from build123d import *

# Parameters (mm, degrees)
BOSS_EXTRUDE1_DEPTH = 3
SKETCH2_R           = 1.5
CUT_EXTRUDE1_DEPTH  = 3
CUT_EXTRUDE2_DEPTH  = 3
SKETCH5_W           = 18
SKETCH5_H           = 3
CUT_EXTRUDE3_DEPTH  = 3
CUT_EXTRUDE5_DEPTH  = 3


with BuildPart() as part:
    # Sketch1 → Boss-Extrude1 (new body)
    with BuildSketch(Plane.XY):
        with BuildLine():
            Line((3.868741846, 4.666984775), (3.868741846, -4.333015225))
            ThreePointArc((3.868741846, -4.333015225), (2.990062189, -6.454335569), (0.868741846, -7.333015225))
            Line((0.868741846, -7.333015225), (-29.131258154, -7.333015225))
            ThreePointArc((-29.131258154, -7.333015225), (-39.055484202, 1.438271074), (-31.570064658, 12.365037303))
            Line((-31.570064658, 12.365037303), (-13.143764854, 16.998769659))
            ThreePointArc((-13.143764854, 16.998769659), (-7.545321729, 14.563041923), (-8.476085741, 8.52905374))
            ThreePointArc((-8.476085741, 8.52905374), (-8.5954965, 7.981289437), (-8.131258154, 7.666984775))
            Line((-8.131258154, 7.666984775), (0.868741846, 7.666984775))
            ThreePointArc((0.868741846, 7.666984775), (2.990062189, 6.788305118), (3.868741846, 4.666984775))
        make_face()
    extrude(amount=BOSS_EXTRUDE1_DEPTH)

    # Sketch2 → Cut-Extrude1 (cut)
    with BuildSketch(Plane.XY.offset(3)):
        with Locations((-29.131258154, 2.666984775)):
            Circle(SKETCH2_R)
    extrude(amount=-CUT_EXTRUDE1_DEPTH, mode=Mode.SUBTRACT)

    # Sketch4 → Cut-Extrude2 (cut)
    with BuildSketch(Plane(origin=(0, 0, 0), x_dir=(-1, 0, 0), z_dir=(0, 0, -1))):
        with BuildLine():
            Line((30.632745307, 6.129616333), (16.185458015, 12.394336069))
            ThreePointArc((16.185458015, 12.394336069), (13.596850059, 11.433034125), (14.450350699, 8.806909749))
            Line((14.450350699, 8.806909749), (26.890771517, -0.370201523))
            ThreePointArc((26.890771517, -0.370201523), (32.402104849, 0.783943915), (30.632745307, 6.129616333))
        make_face()
    extrude(amount=-CUT_EXTRUDE2_DEPTH, mode=Mode.SUBTRACT)

    # Sketch5 → Cut-Extrude3 (cut)
    with BuildSketch(Plane.XY.offset(3)):
        with Locations((-8.131258154, -1.533015225)):
            Rectangle(SKETCH5_W, SKETCH5_H)
    extrude(amount=-CUT_EXTRUDE3_DEPTH, mode=Mode.SUBTRACT)

    # Sketch7 → Cut-Extrude5 (cut)
    with BuildSketch(Plane.XY.offset(3)):
        with BuildLine():
            Line((-14.631258154, -0.033015225), (-14.631258154, 3.966984775))
            ThreePointArc((-14.631258154, 3.966984775), (-14.338364936, 4.674091556), (-13.631258154, 4.966984775))
            Line((-13.631258154, 4.966984775), (-2.631258154, 4.966984775))
            ThreePointArc((-2.631258154, 4.966984775), (-1.924151373, 4.674091556), (-1.631258154, 3.966984775))
            Line((-1.631258154, 3.966984775), (-1.631258154, -0.033015225))
            Line((-1.631258154, -0.033015225), (-14.631258154, -0.033015225))
        make_face()
    extrude(amount=-CUT_EXTRUDE5_DEPTH, mode=Mode.SUBTRACT)


solid = part.part
Verification items for the finished model (mm, model axes). A direction names the side the tool comes from. Coordinates: 2 decimals unless noted, no trailing zeros. Order: outer loops, then holes, each group sorted by start corner. A loop starts at its lowest first (then second) coordinate and runs counter-clockwise, first axis right, second up. Notation, with made-up numbers: (74, -10) -> (86, -10) arc R16 ccw to (86, 20) -> close; hole circle Ø3 at (0.5, 37.25). An arc over 180 degrees is marked (long way). Put each result on its own line as item: value. Start each with the question number.
1. Go/stop test with flat-tipped pins: pin 1 Ø12 at (x, y) = (-29.13, 2.67) entering from -Z; pin 2 Ø1.5 at (x, z) = (-4, 1.5) entering from +Y. Record where each tip stops, or that it passes through.
2. Mould release check, pull along X, two halves, no side actions. Record for faces 3 (the flat face through (-17, 2, 3)), 4 (the flat face through (-14.631, 2, 2)), 5 (the flat face through (3.869, 0, 1)): released by +X, released by -X, zero draft, split by the parting line, or undercut.
3. Cross-section at D-D, the plane y = 1. Record the boundary of the cut face in (x, z), then the cut area to 3 significant figures.
4. Cross-section at A-A, the plane x = -21.5. Record the boundary of the cut face in (y, z).
5. Access from +Z, -Z, +X, -X, +Y, -Y to the whole of each face (thin tool, end or side, straight path). Record for faces 1 (the flat face through (-17.131, -2, 2)), 2 (the flat face through (-17, 2, 0)).
6. Material ranges on L1, parallel to Y at x = 0.5, z = 1.9; L2, parallel to X at y = 4.5, z = 2; L3, parallel to Y at x = -8.5, z = 2.5, recorded low to high. Write a range as [from, to].
7. Cross-section at B-B, the plane y = 10.5. Record the boundary of the cut face in (x, z).
8. Cross-section at C-C, the plane x = -15.5. Record the boundary of the cut face in (y, z).
Computed:
1. pin 1: z = 0
1. pin 2: y = 7.67
2. face 3: zero draft
2. face 4: undercut
2. face 5: released by +X
3. outline: (-38.99, 0) -> (-32.52, 0) -> (-32.52, 3) -> (-38.99, 3) -> close; (-25.03, 0) -> (-14.63, 0) -> (-14.63, 3) -> (-25.03, 3) -> close; (-1.63, 0) -> (3.87, 0) -> (3.87, 3) -> (-1.63, 3) -> close
3. area: 67.1 mm2
4. outline: (-7.33, 0) -> (3.61, 0) -> (3.61, 3) -> (-7.33, 3) -> close; (10.09, 0) -> (14.9, 0) -> (14.9, 3) -> (10.09, 3) -> close
5. face 1: +Z, -Z
5. face 2: -Z, +X, -X, +Y, -Y
6. L1: [-7.33, -3.03], [-0.03, 7.67]
6. L2: [-38.96, -32.43], [-20.29, -14.48], [-1.79, 3.87]
6. L3: [-7.33, -3.03], [4.97, 7.83], [8.5, 15.79]
7. outline: (-35.35, 0) -> (-20.55, 0) -> (-20.55, 3) -> (-35.35, 3) -> close; (-13.4, 0) -> (-7.2, 0) -> (-7.2, 3) -> (-13.4, 3) -> close
8. outline: (-7.33, 0) -> (-3.03, 0) -> (-3.03, 3) -> (-7.33, 3) -> close; (-0.03, 0) -> (8.03, 0) -> (8.03, 3) -> (-0.03, 3) -> close; (12.56, 0) -> (16.41, 0) -> (16.41, 3) -> (12.56, 3) -> close
